```python
from build123d import *

# Parameters (mm, degrees)
F1_DEPTH = 6.35


with BuildPart() as f1:
    # F0 (on Top) → F1 (new body)
    with BuildSketch(Plane.XY):
        Polygon((-139.7, 0), (0, 0), (139.7, 0), (139.7, 76.2), (300.026565, 507.997021), (19.052757, 507.997021), (19.05, 507.997021), (19.446046, 504.696671), (57.15, 190.5), (16.933333, 152.4), (0, 152.4), (-16.932315, 152.4), (-57.15, 190.5), (-19.05, 507.998044), (-300.023808, 507.998044), (-139.7, 76.2), align=None)
        with BuildLine():
            ThreePointArc((9.525, 127), (6.735192, 120.264808), (0, 117.475))
            ThreePointArc((0, 117.475), (-6.735192, 133.735192), (9.525, 127))
        make_face(mode=Mode.SUBTRACT)
    extrude(amount=F1_DEPTH)


solid = f1.part
```
Here's how the part is built. I have some questions about the finished solid (model axes, mm). A direction names the side the tool comes from. Give positions to 0.01 mm unless a question says otherwise; leave off trailing zeros. Loops run counter-clockwise (first coordinate to the right, second up) from the corner with the lowest first, then second, coordinate; pieces in that order, holes last. Notation, with made-up numbers: M 76,22.25 L 118,22.25 A11 cw 118,40.25 Z; hole C 35.5,13.25 d1. An arc over 180 degrees is marked long. Return JSON: item names as keys, results as strings.
Item 1: I'm going to push flat-ended pins straight in: pin 1 Ø1.5 at (y, z) = (385, 5.5) entering from +X; pin 2 Ø1.9 at (y, z) = (36, 2) entering from +X; pin 3 Ø3 at (x, z) = (-7, 4.5) entering from +Y. Where does each tip first touch, or does it pass through?
A:
{"pin 1": "stops at x = 254.64", "pin 2": "stops at x = 139.7", "pin 3": "stops at y = 152.4"}
Item 2: Imagine slicing it at C-C on x = 45. List the corners of the cut face in (y, z) for me, then the cut area to 3 significant figures.
A:
{"outline": "M 0,0 L 178.99,0 L 178.99,6.35 L 0,6.35 Z; M 291.75,0 L 508,0 L 508,6.35 L 291.75,6.35 Z", "area": "2,510 mm^2"}
Item 3: Please list where these lines run through material, in increasing order: line 1 (Y direction, x = 0, z = 2) (3 decimals); line 2 (Y direction, x = 119, z = 3.5); line 3 (X direction, y = 172.5, z = 2.5).
A:
{"line 1": "y = 0 to 117.475, 136.525 to 152.4", "line 2": "y = 0 to 508", "line 3": "x = -175.46 to -38.15, 38.15 to 175.46"}
Item 4: On a 3-axis mill with a long thin cutter (end or side, diameter ignored), from which of +Z, -Z, +X, -X, +Y, -Y can I reach the whole of each face in a straight line? I mean faces 1 (the flat face through (-36.76, 171.183, 3.131)), 2 (the flat face through (218.741, 289.076, 3.131)). Say none if no direction works.
A:
{"face 1": "+Z, -Z", "face 2": "+Z, -Z, +X, -Y"}
Item 5: Imagine slicing it at D-D on y = 68. List the corners of the cut face in (x, z) for me.
A:
{"outline": "M -139.7,0 L 139.7,0 L 139.7,6.35 L -139.7,6.35 Z"}
Item 6: Imagine slicing it at B-B on y = 215. List the corners of the cut face in (x, z) for me.
A:
{"outline": "M -191.24,0 L -54.21,0 L -54.21,6.35 L -191.24,6.35 Z; M 54.21,0 L 191.24,0 L 191.24,6.35 L 54.21,6.35 Z"}
Item 7: Thinking about a two-plate mould opening in Y: for faces 3 (the flat face through (62, 258, 6.35)), 4 (the flat face through (-38.367, 347.027, 3.131)), 5 (the flat face through (-220.984, 295.122, 3.131)), which applies, released by +Y, released by -Y, zero draft, split by the parting line, or undercut?
A:
{"face 3": "zero draft", "face 4": "undercut", "face 5": "released by -Y"}
Item 8: Imagine slicing it at A-A on z = 5. List the corners of the cut face in (x, y) for me (3 decimals), then the cut area to 3 significant figures.
A:
{"outline": "M -300.024,507.998 L -139.7,76.2 L -139.7,0 L 139.7,0 L 139.7,76.2 L 300.027,507.997 L 19.05,507.997 L 57.15,190.5 L 16.933,152.4 L -16.932,152.4 L -57.15,190.5 L -19.05,507.998 Z; hole C 0,127 d19.05", "area": "184,000 mm^2"}
